Verification items for this drawing (mm, ordinates from the low corner). A direction names the side the tool comes from. Round coordinates to 2 decimals unless told otherwise and drop trailing zeros. Loops run counter-clockwise (first coordinate to the right, second up) from the corner with the lowest first, then second, coordinate; pieces in that order, holes last. Notation, with made-up numbers: (10.5, -29.75) - (16.5, -29.75) arc R20 cw to (16.5, -9.75) - close; hole circle Ø5 at (-33.5, 89.5). An arc over 180 degrees is marked (long way). Use a Markdown table: item, result. Add a question column.
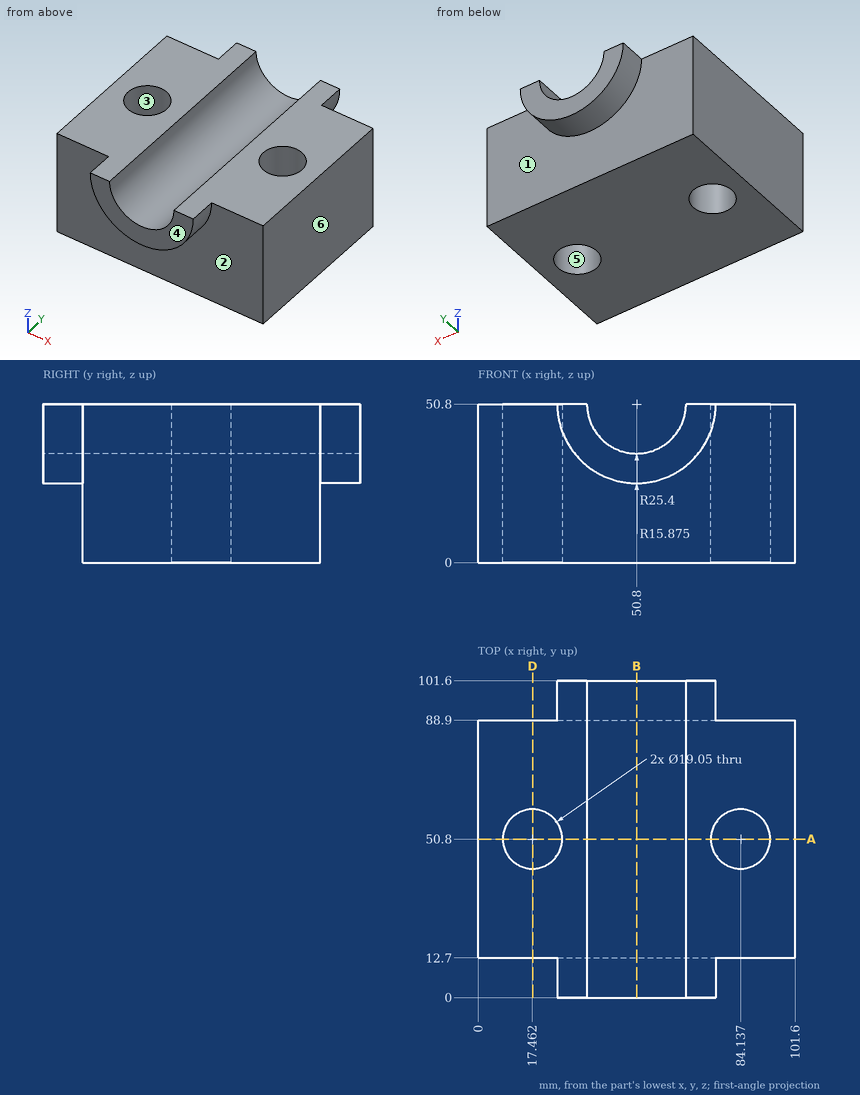
Q1. Go/stop test with flat-tipped pins: pin 1 Ø1.5 at (y, z) = (47, 22) entering from -X; pin 2 Ø6 at (x, z) = (15.5, 35) entering from -Y. Record where each tip stops, or that it passes through.
Q2. Set-up check for the marked faces 1, 2 and 3: record each of +Z, -Z, +X, -X, +Y, -Y from which the full face is reachable in a straight line by a thin tool's end or side.
Q3. Thickness scan on line 1 along X through (y, z) = (49, 23.5) (1 decimal); line 2 along Y through (x, z) = (97, 24); line 3 along Y through (x, z) = (14, 44.5) (1 decimal). Record the ranges inside material, lowest first.
Q4. Release check for a two-part mould opening along Y. For the marked faces 4, 5 and 6 record: +Y half, -Y half, draft (parallel to the pull), parting line (faces both ways), or undercut.
Q5. Section check A-A on y = 50.8. State how many separate pieces and enclosed holes the cut face has, plus the area to 3 significant figures.
Q6. Section check B-B on x = 50.8. Record the cut outline in (y, z) (1 decimal), plus the area to 3 significant figures.
Q7. Section check D-D on x = 17.5. Record the cut outline in (y, z) (1 decimal).
Determined:
| question | item | result |
|---|---|---|
| 1 | pin 1 | stops at x = 0 |
| 1 | pin 2 | stops at y = 12.7 |
| 2 | face 1 | -Z, +Y |
| 2 | face 2 | -Z, -Y |
| 2 | face 3 | +Z, -Z |
| 3 | line 1 | x = 0 to 8.1, 26.8 to 74.8, 93.5 to 101.6 |
| 3 | line 2 | y = 12.7 to 88.9 |
| 3 | line 3 | y = 12.7 to 41.9, 59.7 to 88.9 |
| 4 | face 4 | -Y half |
| 4 | face 5 | undercut |
| 4 | face 6 | draft |
| 5 | separate pieces | 3 |
| 5 | enclosed holes | 0 |
| 5 | area | 2,830 mm² |
| 6 | outline | (0, 25.4) - (12.7, 25.4) - (12.7, 0) - (88.9, 0) - (88.9, 25.4) - (101.6, 25.4) - (101.6, 34.9) - (0, 34.9) - close |
| 6 | area | 2,900 mm² |
| 7 | outline | (12.7, 0) - (41.3, 0) - (41.3, 50.8) - (12.7, 50.8) - close; (60.3, 0) - (88.9, 0) - (88.9, 50.8) - (60.3, 50.8) - close |
